Answer from the drawing. Dimensions are ordinates in mm from the lowest x, y and z of the part. Give positions to 0.01 mm unless a question says otherwise; leave off trailing zeros. Write each loop counter-clockwise with the first axis right and the second up, starting at its lowest first coordinate (ties: lowest second). Pieces come first, ordered by that corner, then holes. Notation, with made-up numbers: M -0.5,-5 L 29.5,-5 A13 ccw 29.5,0 Z; hole C -21,32.25 d7. An arc over 180 degrees is marked long. Put each result on its own line as item: value.
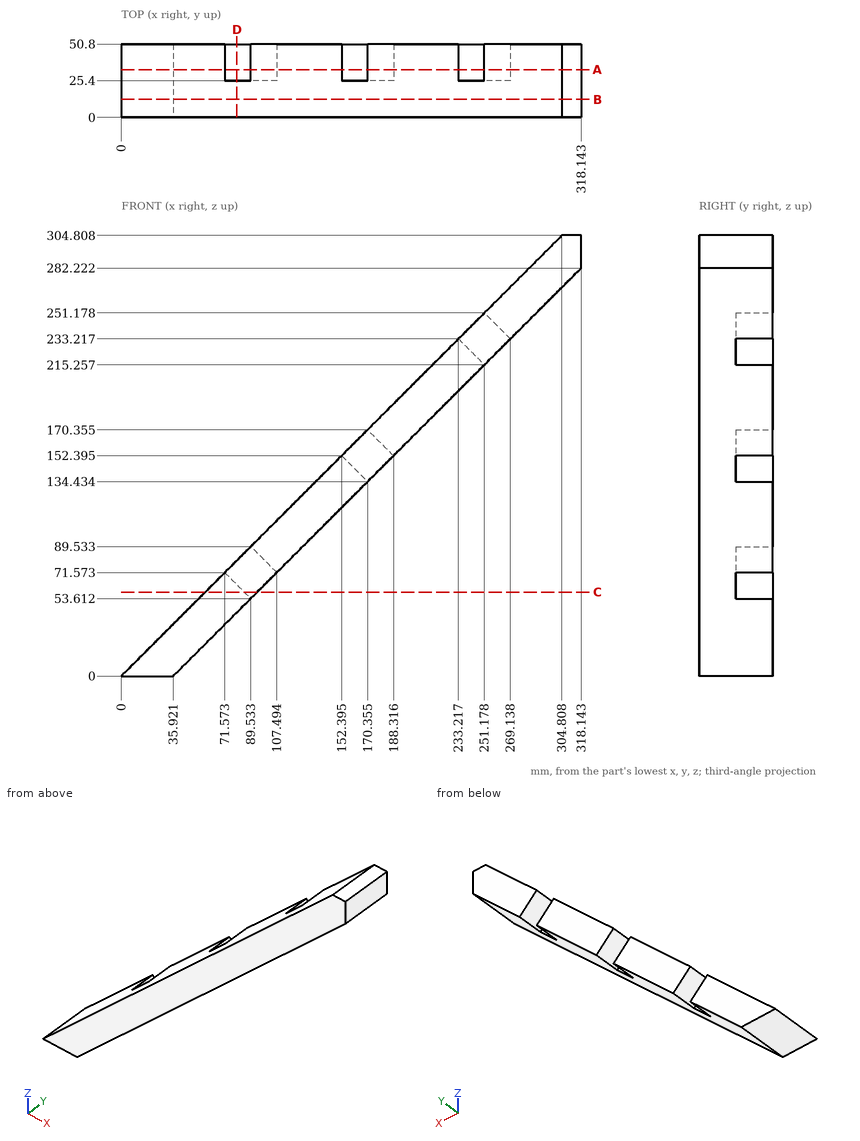
(1) Section D-D on x = 80 is taken. Determine the outline of the cut face in (y, z) (1 decimal).
Result:
outline: M 0,44.1 L 50.8,44.1 L 50.8,63.1 L 25.4,63.1 L 25.4,80 L 0,80 Z
(2) Given pin 1 Ø1.5 at (y, z) = (32.5, 131) entering from -X; pin 2 Ø5 at (x, y) = (174, 7) entering from +Z; pin 3 Ø1.5 at (y, z) = (35.5, 150.5) entering from -X, each flat-ended and moving along its own axis, determine where each tip first touches the part or whether it passes through.
Result:
pin 1: stops at x = 130.25
pin 2: stops at z = 176.5
pin 3: stops at x = 149.75
(3) Straight lines are drawn through the part: line 1 along X through (y, z) = (22, 81); line 2 along Z through (x, y) = (277.5, 9); line 3 along X through (y, z) = (15, 21.5). For each, find the intervals that lie inside material, in ascending order. Write a range as from..to.
Result:
line 1: x = 81..116.92
line 2: z = 241.58..277.5
line 3: x = 21.5..57.42
(4) Section A-A on y = 33 is taken. Determine the outline of the cut face in (x, z) (1 decimal).
Result:
outline: M 0,0 L 35.9,0 L 89.5,53.6 L 71.6,71.6 Z; M 89.5,89.5 L 107.5,71.6 L 170.4,134.4 L 152.4,152.4 Z; M 170.4,170.4 L 188.3,152.4 L 251.2,215.3 L 233.2,233.2 Z; M 251.2,251.2 L 269.1,233.2 L 318.1,282.2 L 318.1,304.8 L 304.8,304.8 Z
(5) Section C-C on z = 58 is taken. Determine the outline of the cut face in (x, y) (1 decimal).
Result:
outline: M 58,0 L 93.9,0 L 93.9,25.4 L 85.1,25.4 L 85.1,50.8 L 58,50.8 Z
(6) Section B-B on y = 12.5 is taken. Determine the outline of the cut face in (x, z).
Result:
outline: M 0,0 L 35.92,0 L 318.14,282.22 L 318.14,304.81 L 304.81,304.81 Z
